For this review, take the finished solid that the model builds, in its own axes (mm). Coordinates: 2 decimals unless noted, no trailing zeros. Write each loop counter-clockwise with the first axis right and the second up, starting at its lowest first coordinate (ties: lowest second). Pieces come first, ordered by that corner, then holes. Notation, with made-up numbers: M 66,61 L 83,61 A15 ccw 83,79 Z; hole C -38,-10.75 d7. An arc over 180 degrees is marked long. Return JSON: item names as keys, results as strings.
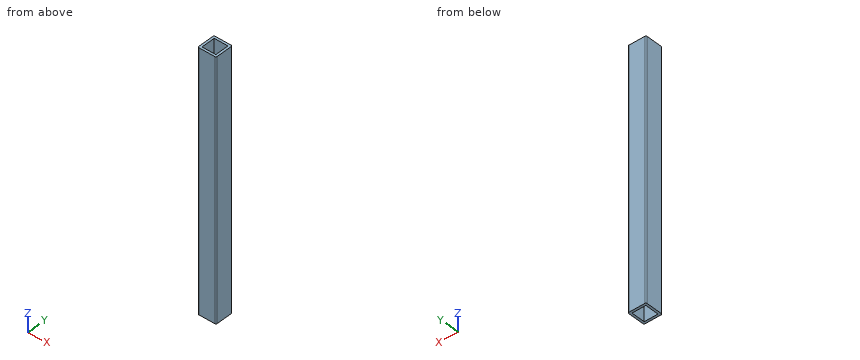
```python
from build123d import *

# Parameters (mm, degrees)
BOSS_EXTRUDE1_DEPTH      = 88.9
BOSS_EXTRUDE1_DEPTH_BACK = 88.9
SKETCH1_W                = 12.7
SKETCH1_H                = 12.7
SKETCH1_W_2              = 9.525
SKETCH1_H_2              = 9.525
FILLET1_R                = 0.79375


with BuildPart() as part:
    # Sketch1 → Boss-Extrude1 (new, two sides: drawn at the far end of the back side and taken through both)
    with BuildSketch(Plane.XY.offset(-BOSS_EXTRUDE1_DEPTH_BACK)):
        Rectangle(SKETCH1_W, SKETCH1_H)
        Rectangle(SKETCH1_W_2, SKETCH1_H_2, mode=Mode.SUBTRACT)
    extrude(amount=BOSS_EXTRUDE1_DEPTH + BOSS_EXTRUDE1_DEPTH_BACK)

    # Fillet1
    fillet1_edges = [part.edges().sort_by_distance(p)[0] for p in [
        (6.35, -6.35, 0),
        (-6.35, -6.35, 0),
        (-6.35, 6.35, 0),
        (6.35, 6.35, 0),
    ]]
    fillet(fillet1_edges, radius=FILLET1_R)


solid = part.part
```
1. Wall thickness on L1, parallel to Y at x = -3.5, z = 78.5; L2, parallel to Y at x = -6, z = 24: over which ranges is each line inside the solid? List them lowest first. Write a range as from..to.
Checks:
{"L1": "-6.35..-4.76, 4.76..6.35", "L2": "-6.21..6.21"}
2. We need section C-C (z = -69). State the section outline as (x, y) points.
Checks:
{"outline": "M -6.35,-5.56 A0.79 ccw -5.56,-6.35 L 5.56,-6.35 A0.79 ccw 6.35,-5.56 L 6.35,5.56 A0.79 ccw 5.56,6.35 L -5.56,6.35 A0.79 ccw -6.35,5.56 Z; hole M -4.76,-4.76 L 4.76,-4.76 L 4.76,4.76 L -4.76,4.76 Z"}
3. We need section A-A (x = -0.75). State the section outline as (y, z) points.
Checks:
{"outline": "M -6.35,-88.9 L -4.76,-88.9 L -4.76,88.9 L -6.35,88.9 Z; M 4.76,-88.9 L 6.35,-88.9 L 6.35,88.9 L 4.76,88.9 Z"}
4. Clearance check with a flat-ended pin moving along its axis: pin 1 Ø6 at (x, y) = (-1, -0.5) entering from +Z. State where the tip first meets the part, or that it passes through.
Checks:
{"pin 1": "through"}
